Can you work these out from the model? Positions are in its coordinate system, mm. A direction names the side the tool comes from. Give positions to 0.01 mm unless a question says otherwise; leave off trailing zeros. Loops run counter-clockwise (first coordinate to the right, second up) from the corner with the lowest first, then second, coordinate; pieces in that order, holes last. Notation, with made-up numbers: (77, 44.25) - (122, 44.25) arc R38 ccw to (122, 83.25) - close; hole circle Ø5 at (17.5, 66). An arc over 180 degrees is marked (long way). Answer as a JSON object with one key per item and string values.
```python
from build123d import *

# Parameters (mm, degrees)
M2_CLEARANCE_HOLE1_D = 2.6
CUT_EXTRUDE1_START   = -5.0000001
CUT_EXTRUDE1_DEPTH   = 5.0000001
CHAMFER1_SIZE        = 1


# Read off the part's stored shape, not the designer's step: Cut-Extrude1
with BuildPart() as part:
    # Sketch1 → Revolve1 (revolve)
    with BuildSketch(Plane.XY, mode=Mode.PRIVATE) as revolve1_sk:
        with BuildLine():
            Line((-0.1384665388769202, 3.8749999999999973), (8.66153346112308, 3.8749999999999982))
            ThreePointArc((8.66153346112308, 3.8749999999999982), (10.075747023496175, 3.289213562373093), (10.661533461123081, 1.874999999999998))
            Line((10.661533461123081, 1.874999999999998), (10.661533461123081, -7.125000000000003))
            Line((10.661533461123081, -7.125000000000003), (13.66153346112308, -7.125000000000003))
            Line((13.66153346112308, -7.125000000000003), (13.661533461123074, -5.524999999999995))
            ThreePointArc((13.661533461123074, -5.524999999999995), (12.323383778668454, -2.9710498941515384), (11.86153346112308, -0.12500000000000358))
            ThreePointArc((11.86153346112308, -0.12500000000000358), (12.323383778668454, 2.721049894151534), (13.661533461123074, 5.274999999999989))
            Line((13.661533461123074, 5.274999999999989), (13.66153346112308, 6.874999999999997))
            Line((13.66153346112308, 6.874999999999997), (-0.1384665388769206, 6.874999999999996))
            Line((-0.1384665388769206, 6.874999999999996), (-0.1384665388769202, 3.8749999999999973))
        make_face()
    revolve(revolve1_sk.sketch.rotate(Axis((-1.3384665388769221, 6.874999999999996, 0), (0, -1, 0)), 90), axis=Axis((-1.3384665388769221, 6.874999999999996, 0), (0, -1, 0)))

    # M2 Clearance Hole1 (through all)
    with Locations(Plane(origin=(0, 6.8749999999999964, 0), x_dir=(1, 3e-17, 0), z_dir=(-3e-17, 1, 0))):
        with Locations((-5.838466539, 0), (-1.338466539, 4.5), (3.161533461, 0), (-1.338466539, -4.5)):
            Hole(M2_CLEARANCE_HOLE1_D / 2)

    # Cut-Extrude1 outline → Cut-Extrude1 (cut)
    with BuildSketch(Plane(origin=(0, 6.8749999999999964, 0), x_dir=(1, 3e-17, 0), z_dir=(-3e-17, 1, 0)).offset(CUT_EXTRUDE1_START)):
        with BuildLine():
            ThreePointArc((10.486994905, -2.039230647), (10.661533461, 0), (10.486994905, 2.039230647))
            ThreePointArc((10.486994905, 2.039230647), (10.040427521, 2.711672352), (9.24272074, 2.835220586))
            Line((9.24272074, 2.835220586), (6.373832713, 2.066504356))
            ThreePointArc((6.373832713, 2.066504356), (6.078257545, 1.846957489), (6.013135437, 1.484570103))
            ThreePointArc((6.013135437, 1.484570103), (6.161533461, 0), (6.013135437, -1.484570103))
            ThreePointArc((6.013135437, -1.484570103), (6.078257545, -1.846957489), (6.373832713, -2.066504356))
            Line((6.373832713, -2.066504356), (9.24272074, -2.835220586))
            ThreePointArc((9.24272074, -2.835220586), (10.040427521, -2.711672352), (10.486994905, -2.039230647))
        make_face()
        with BuildLine():
            ThreePointArc((8.148366442, 5.477225575), (8.625068522, 6.128651244), (8.465351258, 6.919910159))
            ThreePointArc((8.465351258, 6.919910159), (7.146814835, 8.485281374), (5.58144362, 9.803817797))
            ThreePointArc((5.58144362, 9.803817797), (4.790184705, 9.963535061), (4.138759036, 9.486832981))
            Line((4.138759036, 9.486832981), (1.149002054, 4.308421985))
            ThreePointArc((1.149002054, 4.308421985), (1.093178843, 3.953353196), (1.289966626, 3.652579786))
            ThreePointArc((1.289966626, 3.652579786), (1.843513976, 3.181980515), (2.314113248, 2.628433165))
            ThreePointArc((2.314113248, 2.628433165), (2.614886658, 2.431645382), (2.969955446, 2.487468593))
            Line((2.969955446, 2.487468593), (8.148366442, 5.477225575))
        make_face()
        with BuildLine():
            ThreePointArc((5.58144362, -9.803817797), (7.146814835, -8.485281374), (8.465351258, -6.919910159))
            ThreePointArc((8.465351258, -6.919910159), (8.625068522, -6.128651244), (8.148366442, -5.477225575))
            Line((8.148366442, -5.477225575), (2.969955446, -2.487468593))
            ThreePointArc((2.969955446, -2.487468593), (2.614886658, -2.431645382), (2.314113248, -2.628433165))
            ThreePointArc((2.314113248, -2.628433165), (1.843513976, -3.181980515), (1.289966626, -3.652579786))
            ThreePointArc((1.289966626, -3.652579786), (1.093178843, -3.953353196), (1.149002054, -4.308421985))
            Line((1.149002054, -4.308421985), (4.138759036, -9.486832981))
            ThreePointArc((4.138759036, -9.486832981), (4.790184705, -9.963535061), (5.58144362, -9.803817797))
        make_face()
        with BuildLine():
            ThreePointArc((1.496754047, 10.581187279), (1.373205813, 11.37889406), (0.700764108, 11.825461444))
            ThreePointArc((0.700764108, 11.825461444), (-1.338466539, 12), (-3.377697186, 11.825461444))
            ThreePointArc((-3.377697186, 11.825461444), (-4.050138891, 11.37889406), (-4.173687125, 10.581187279))
            Line((-4.173687125, 10.581187279), (-3.404970895, 7.712299252))
            ThreePointArc((-3.404970895, 7.712299252), (-3.185424028, 7.416724084), (-2.823036642, 7.351601976))
            ThreePointArc((-2.823036642, 7.351601976), (-1.338466539, 7.5), (0.146103564, 7.351601976))
            ThreePointArc((0.146103564, 7.351601976), (0.50849095, 7.416724084), (0.728037817, 7.712299252))
            Line((0.728037817, 7.712299252), (1.496754047, 10.581187279))
        make_face()
        with BuildLine():
            ThreePointArc((-3.377697186, -11.825461444), (-1.338466539, -12), (0.700764108, -11.825461444))
            ThreePointArc((0.700764108, -11.825461444), (1.373205813, -11.37889406), (1.496754047, -10.581187279))
            Line((1.496754047, -10.581187279), (0.728037817, -7.712299252))
            ThreePointArc((0.728037817, -7.712299252), (0.50849095, -7.416724084), (0.146103564, -7.351601976))
            ThreePointArc((0.146103564, -7.351601976), (-1.338466539, -7.5), (-2.823036642, -7.351601976))
            ThreePointArc((-2.823036642, -7.351601976), (-3.185424028, -7.416724084), (-3.404970895, -7.712299252))
            Line((-3.404970895, -7.712299252), (-4.173687125, -10.581187279))
            ThreePointArc((-4.173687125, -10.581187279), (-4.050138891, -11.37889406), (-3.377697186, -11.825461444))
        make_face()
        with BuildLine():
            ThreePointArc((-6.815692114, 9.486832981), (-7.467117783, 9.963535061), (-8.258376698, 9.803817797))
            ThreePointArc((-8.258376698, 9.803817797), (-9.823747913, 8.485281374), (-11.142284336, 6.919910159))
            ThreePointArc((-11.142284336, 6.919910159), (-11.3020016, 6.128651244), (-10.825299519, 5.477225575))
            Line((-10.825299519, 5.477225575), (-5.646888524, 2.487468593))
            ThreePointArc((-5.646888524, 2.487468593), (-5.291819735, 2.431645382), (-4.991046325, 2.628433165))
            ThreePointArc((-4.991046325, 2.628433165), (-4.520447054, 3.181980515), (-3.966899704, 3.652579786))
            ThreePointArc((-3.966899704, 3.652579786), (-3.770111921, 3.953353196), (-3.825935132, 4.308421985))
            Line((-3.825935132, 4.308421985), (-6.815692114, 9.486832981))
        make_face()
        with BuildLine():
            ThreePointArc((-11.142284336, -6.919910159), (-9.823747913, -8.485281374), (-8.258376698, -9.803817797))
            ThreePointArc((-8.258376698, -9.803817797), (-7.467117783, -9.963535061), (-6.815692114, -9.486832981))
            Line((-6.815692114, -9.486832981), (-3.825935132, -4.308421985))
            ThreePointArc((-3.825935132, -4.308421985), (-3.770111921, -3.953353196), (-3.966899704, -3.652579786))
            ThreePointArc((-3.966899704, -3.652579786), (-4.520447054, -3.181980515), (-4.991046325, -2.628433165))
            ThreePointArc((-4.991046325, -2.628433165), (-5.291819735, -2.431645382), (-5.646888524, -2.487468593))
            Line((-5.646888524, -2.487468593), (-10.825299519, -5.477225575))
            ThreePointArc((-10.825299519, -5.477225575), (-11.3020016, -6.128651244), (-11.142284336, -6.919910159))
        make_face()
        with BuildLine():
            ThreePointArc((-11.919653818, 2.835220586), (-12.717360599, 2.711672352), (-13.163927983, 2.039230647))
            ThreePointArc((-13.163927983, 2.039230647), (-13.338466539, 0), (-13.163927983, -2.039230647))
            ThreePointArc((-13.163927983, -2.039230647), (-12.717360599, -2.711672352), (-11.919653818, -2.835220586))
            Line((-11.919653818, -2.835220586), (-9.05076579, -2.066504356))
            ThreePointArc((-9.05076579, -2.066504356), (-8.755190623, -1.846957489), (-8.690068515, -1.484570103))
            ThreePointArc((-8.690068515, -1.484570103), (-8.838466539, 0), (-8.690068515, 1.484570103))
            ThreePointArc((-8.690068515, 1.484570103), (-8.755190623, 1.846957489), (-9.05076579, 2.066504356))
            Line((-9.05076579, 2.066504356), (-11.919653818, 2.835220586))
        make_face()
    extrude(amount=CUT_EXTRUDE1_DEPTH, mode=Mode.SUBTRACT)

    # Chamfer1
    chamfer1_edges = [part.edges().sort_by_distance(p)[0] for p in [
        (-1.3384665388769197, -7.125000000000003, -12.000000000000004),
    ]]
    chamfer(chamfer1_edges, length=CHAMFER1_SIZE)


solid = part.part
```
1) Imagine slicing it at C-C on y = -4.25. Write out the boundary of the cut face in (x, z).
Check sheet entries:
{"outline": "circle Ø28.4 at (-1.34, 0); hole circle Ø24 at (-1.34, 0)"}
2) Imagine slicing it at D-D on y = 0. Write out the boundary of the cut face in (x, z).
Check sheet entries:
{"outline": "circle Ø26.4 at (-1.34, 0); hole circle Ø24 at (-1.34, 0)"}
3) Which directions (+Z, -Z, +X, -X, +Y, -Y) give clear straight access to the entire face, cutting with the end or side of a thin tool? Please do faces 3 (the cylindrical face through (4.78, 4.9, 9.96)), 4 (the flat face through (-2, 6.875, 3)).
Check sheet entries:
{"face 3": "+Y, -Y", "face 4": "+Z, -Z, +X, -X, +Y"}
4) Imagine slicing it at A-A on z = 0. Give the number of separate pieces and of enclosed holes in the cut face, and give its area (3 significant figures).
Check sheet entries:
{"separate pieces": "6", "enclosed holes": "0", "area": "78.7 mm2"}
5) If we mould it in two halves opening along Z, with no side actions, what happens to faces 1 (the flat face through (-3.784, 5.231, 9.127)), 2 (the flat face through (-14, -7.125, 5))? For each: released by +Z, released by -Z, zero draft, split by the parting line, or undercut.
Check sheet entries:
{"face 1": "undercut", "face 2": "zero draft"}
6) I'm going to push flat-ended pins straight in: P1, Ø2.5, axis at x = -1.34, z = 4.5, coming from the -Y side; P2, Ø1, axis at x = 9.5, y = 4, coming from the +Z side; P3, Ø4, axis at x = -10.5, z = 5, coming from the -Y side; P4, Ø6, axis at x = -3.5, z = -1.5, coming from the -Y side (3 decimals). Where does each tip first touch, or does it pass through?
Check sheet entries:
{"P1": "through", "P2": "z = 9.87", "P3": "y = -6.56", "P4": "y = 3.875"}
7) I need wall thicknesses on L1, parallel to X at y = 4, z = 7; L2, parallel to Z at x = -6.5, y = 6; L3, parallel to X at y = 5.35, z = -4.5. Which ranges of each line are inside material? Lowest first, please.
Check sheet entries:
{"L1": "-13.69 to -11.09, -5.38 to 2.7, 8.41 to 11.02", "L2": "-14.08 to -8.94, -2.98 to -1.12, 1.12 to 2.98, 8.94 to 14.08", "L3": "-15.65 to -9.13, -3.94 to -2.64, -0.04 to 1.26, 6.46 to 12.97"}
